Answer from the drawing. Dimensions are ordinates in mm from the lowest x, y and z of the part. A direction names the side the tool comes from. Give positions to 0.01 mm unless a question says otherwise; leave off trailing zeros. Write each loop counter-clockwise with the first axis right and the second up, starting at its lowest first coordinate (ties: lowest second). Pieces come first, ordered by that corner, then holes.
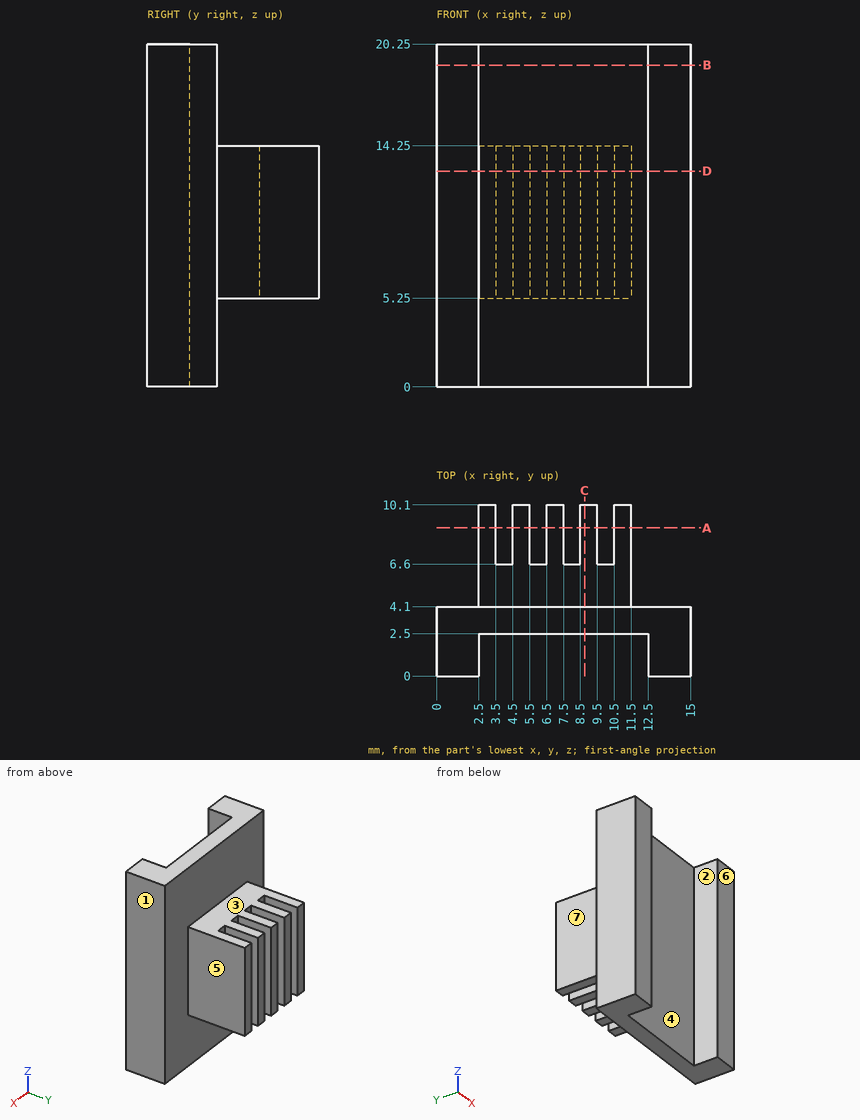
Item 1: A cutting plane is placed at A-A, the plane y = 8.75. Give the vertices of the cut face in (x, z), plus the area to 3 significant figures.
Conclusion:
outline: (2.5, 5.25) - (3.5, 5.25) - (3.5, 14.25) - (2.5, 14.25) - close; (4.5, 5.25) - (5.5, 5.25) - (5.5, 14.25) - (4.5, 14.25) - close; (6.5, 5.25) - (7.5, 5.25) - (7.5, 14.25) - (6.5, 14.25) - close; (8.5, 5.25) - (9.5, 5.25) - (9.5, 14.25) - (8.5, 14.25) - close; (10.5, 5.25) - (11.5, 5.25) - (11.5, 14.25) - (10.5, 14.25) - close
area: 45.0 mm2
Item 2: A cutting plane is placed at B-B, the plane z = 19. Give the vertices of the cut face in (x, y).
Conclusion:
outline: (0, 0) - (2.5, 0) - (2.5, 2.5) - (12.5, 2.5) - (12.5, 0) - (15, 0) - (15, 4.1) - (0, 4.1) - close
Item 3: A cutting plane is placed at D-D, the plane z = 12.75. Give the vertices of the cut face in (x, y).
Conclusion:
outline: (0, 0) - (2.5, 0) - (2.5, 2.5) - (12.5, 2.5) - (12.5, 0) - (15, 0) - (15, 4.1) - (11.5, 4.1) - (11.5, 10.1) - (10.5, 10.1) - (10.5, 6.6) - (9.5, 6.6) - (9.5, 10.1) - (8.5, 10.1) - (8.5, 6.6) - (7.5, 6.6) - (7.5, 10.1) - (6.5, 10.1) - (6.5, 6.6) - (5.5, 6.6) - (5.5, 10.1) - (4.5, 10.1) - (4.5, 6.6) - (3.5, 6.6) - (3.5, 10.1) - (2.5, 10.1) - (2.5, 4.1) - (0, 4.1) - close
Item 4: Each of these flat-tipped pins is pushed along its axis until it touches: P1, Ø5, axis at y = 6, z = 12, coming from the -X side; P2, Ø3, axis at x = 7.5, y = 7, coming from the +Z side; P3, Ø0.5, axis at x = 4, z = 9, coming from the +Y side; P4, Ø1.8, axis at y = 8.5, z = 8, coming from the -X side. Where does it stop, or does it pass through?
Conclusion:
P1: stops at x = 0
P2: stops at z = 14.25
P3: stops at y = 6.6
P4: stops at x = 2.5
Item 5: Which of the six approach directions +Z, -Z, +X, -X, +Y, -Y give full straight-line access (tool end or side, diameter ignored) to the marked faces 5, 6 and 7?
Conclusion:
face 5: +Z, -Z, +X, +Y
face 6: +Z, -Z, +X, -X, -Y
face 7: +Z, -Z, -X, +Y
Item 6: Consider probe 1 along X at (y, z) = (9, 14); probe 2 along X at (y, z) = (1.75, 7.25); probe 3 along Y at (x, z) = (0.5, 6.25). Determine where each line is inside the solid, lowest interval first.
Conclusion:
probe 1: x = 2.5 to 3.5, 4.5 to 5.5, 6.5 to 7.5, 8.5 to 9.5, 10.5 to 11.5
probe 2: x = 0 to 2.5, 12.5 to 15
probe 3: y = 0 to 4.1
Item 7: A cutting plane is placed at C-C, the plane x = 8.75. Give the vertices of the cut face in (y, z), plus the area to 3 significant figures.
Conclusion:
outline: (2.5, 0) - (4.1, 0) - (4.1, 5.25) - (10.1, 5.25) - (10.1, 14.25) - (4.1, 14.25) - (4.1, 20.25) - (2.5, 20.25) - close
area: 86.4 mm2
Item 8: Determine the mould class of the marked faces 1, 2, 3 and 4 for opening direction X: pulls with the +X half, pulls with the -X half, needs draft (parallel to the pull), parting line crosses it, or undercut.
Conclusion:
face 1: pulls with the +X half
face 2: undercut
face 3: needs draft
face 4: undercut
